Autodesk Inventor part; units mm, degrees
ref_plane "YZ Plane" through (0, 0, 0) normal (1, 0, 0) x (0, 1, 0)
ref_plane "XZ Plane" through (0, 0, 0) normal (0, 1, 0) x (-1, 0, 0)
ref_plane "XY Plane" through (0, 0, 0) normal (0, 0, 1) x (1, 0, 0)
sketch "Sketch1" plane through (0, 0, 0) normal (0, 1, 0) x (-1, 0, 0)
  line L0 (6.1765, 12) -> (-98.8235, 12)
  line L1 (-98.8235, 12) -> (-98.8235, -102)
  line L2 (-6.8235, 12) -> (-6.8235, 18)
  line L3 (-6.8235, 18) -> (6.1765, 18)
  line L4 (6.1765, 18) -> (6.1765, 12)
  line L5 (-98.8235, 12) -> (-98.8235, 18)
  line L6 (-98.8235, 18) -> (-85.8235, 18)
  line L7 (-85.8235, 18) -> (-85.8235, 12)
  line L8 (-98.8235, -102) -> (-85.8235, -87.8857)
  line L9 (-6.8235, -2.1143) -> (6.1765, 12)
  line L10 (-98.8235, -102) -> (-80.8235, -102)
  line L11 (6.1765, 12) -> (-80.8235, -102)
  point P0 (0, 0)
  point P1 (-96.8235, 18)
  point P2 (-96.8235, 18)
  dimension "d0" = 114
  dimension "d1" = 105
  dimension "d2" = 13
  dimension "d3" = 6
  dimension "d4" = 13
  dimension "d5" = 6
  dimension "d6" = 18
extrude "Extrusion1" add sketch "Sketch1" along normal blind 2
sketch "Sketch2" plane through (0, 2, 0) normal (0, 1, 0) x (1, 0, 0)
  line L0 (98.8235, 102) -> (80.8235, 102)
  line L1 (95.8235, 102) -> (87.8235, 102)
  line L2 (87.8235, 102) -> (87.8235, 92)
  line L3 (87.8235, 92) -> (95.8235, 92)
  line L4 (95.8235, 92) -> (95.8235, 102)
  line L5 (98.8235, -18) -> (98.8235, 102)
  point P0 (0, 0)
  dimension "d9" = 10
  dimension "d10" = 8
  dimension "d11" = 3
extrude "Extrusion2" add sketch "Sketch2" along normal blind 3
fillet "Fillet1" radius 4 2 edges at (87.8235, 5, -97) (95.8235, 5, -97)
sketch "Sketch3" plane through (0, 0, 0) normal (0, -1, 0) x (1, 0, 0)
  line L0 (87.8235, -102) -> (80.8235, -102)
  line L1 (87.8235, -102) -> (95.8235, -102)
  line L2 (95.8235, -102) -> (95.8235, -92)
  line L3 (95.8235, -92) -> (87.8235, -92)
  line L4 (87.8235, -92) -> (87.8235, -102)
  line L5 (98.8235, 18) -> (98.8235, -102)
  point P0 (0, 0)
  dimension "d16" = 10
  dimension "d17" = 8
  dimension "d18" = 3
extrude "Extrusion3" add sketch "Sketch3" along normal blind 3
fillet "Fillet3" radius 4 2 edges at (87.8235, -3, -97) (95.8235, -3, -97)
sketch "Sketch4" plane through (80.8235, 0, -102) normal (0, 0, -1) x (-1, 0, 0)
  arc A0 (-15, 0) -> (-11.127, -3) centre (-11.127, 1) ccw
  line L0 (-11.127, 4.8105) -> (-11.127, -3)
  circle A1 centre (-11.127, 1) radius 2.5
  point P0 (80.8235, 0)
  dimension "d25" = 5
extrude "Extrusion4" cut sketch "Sketch4" against normal blind 5
sketch "Sketch5" plane through (0, 2, 0) normal (0, 1, 0) x (1, 0, 0)
  line L0 (85.8235, -12) -> (85.8235, -18)
  line L1 (85.8235, -12) -> (98.8235, -12)
  line L2 (98.8235, -18) -> (98.8235, 102)
  circle A0 centre (92.3235, -12) radius 2.5
  point P0 (0, 0)
  dimension "d26" = 5
extrude "Extrusion5" cut sketch "Sketch5" against normal blind 2
sketch "Sketch6" plane through (0, 2, 0) normal (0, 1, 0) x (1, 0, 0)
  line L0 (-6.1765, -12) -> (-6.1765, -18)
  line L1 (6.8235, -18) -> (6.8235, -12)
  line L2 (-6.1765, -12) -> (6.8235, -12)
  circle A0 centre (0.3235, -12) radius 2.5
  point P0 (0, 0)
  dimension "d29" = 5
  dimension "d32" = 6.5
  dimension "d33" = 6
extrude "Extrusion6" cut sketch "Sketch6" against normal blind 2
equation "\"d23\" = d22"
properties part number "Triangle"
Input: part model. Units: mm. Frame: model coordinates. A direction names the side the tool comes from. Coordinates: 2 decimals unless noted, no trailing zeros. Loops run counter-clockwise (first coordinate to the right, second up) from the corner with the lowest first, then second, coordinate; pieces in that order, holes last. Notation, with made-up numbers: (-7, 59) - (36, 59) arc R18 cw to (36, 66) - close; hole circle Ø10 at (8.25, 3). An arc over 180 degrees is marked (long way). Answer in a Markdown table with one row per item. Add a question column.
Item 1: Contact query for flat-ended pins moving along their axis: P1, Ø1.5, axis at x = 90.5, y = 3.5, coming from the +Z side; P2, Ø4, axis at x = 0.32, z = 12, coming from the -Y side; P3, Ø1.5, axis at x = 58, z = -58.5, coming from the -Y side; P4, Ø12, axis at x = 63, z = -82, coming from the +Y side. Output: stop coordinate, or through.
Item 2: Section query A-A on z = -48. Return the cut outline in (x, y), then the cut area to 3 significant figures.
Item 3: Access query for faces 5 (the cylindrical face through (89.22, -2.14, -96.93)), 6 (the flat face through (92, -1, -92)), 7 (the cylindrical face through (89.566, 1.751, -99.535)). Directions: +Z, -Z, +X, -X, +Y, -Y. A direction counts if a zero-diameter tool reaches every point of the face in a straight line with its end or side. Return the directions, or none.
Item 4: Mould query, pull axis Y, two halves, no side actions, for faces 1 (the flat face through (70, 0, -41)), 2 (the cylindrical face through (94.43, 4.14, -96.93)), 3 (the flat face through (92, 3, -92)), 4 (the flat face through (92, 1, -97)). Classes: released by +Y, released by -Y, zero draft, split by the parting line, or undercut.
Item 5: Section query B-B on x = 59.5. Return the cut outline in (y, z), then the cut area to 3 significant figures.
Item 6: Line query: line 1 along Y through (x, z) = (69.5, -55); line 2 along X through (y, z) = (1, -100.15); line 3 along Z through (x, y) = (68.5, 0.75). Output: solid intervals per line, ascending. Write a range as [from, to].
Recorded:
| question | item | result |
|---|---|---|
| 1 | P1 | z = -92 |
| 1 | P2 | through |
| 1 | P3 | y = 0 |
| 1 | P4 | y = 2 |
| 2 | outline | (39.61, 0) - (98.82, 0) - (98.82, 2) - (39.61, 2) - close |
| 2 | area | 118 mm^2 |
| 3 | face 5 | +Z, -Z, -X, -Y |
| 3 | face 6 | +Z, +X, -X, -Y |
| 3 | face 7 | -Z |
| 4 | face 1 | released by -Y |
| 4 | face 2 | released by +Y |
| 4 | face 3 | zero draft |
| 4 | face 4 | undercut |
| 5 | outline | (0, -74.06) - (2, -74.06) - (2, 12) - (0, 12) - close |
| 5 | area | 172 mm^2 |
| 6 | line 1 | [0, 2] |
| 6 | line 2 | [79.41, 89.45], [94.45, 98.82] |
| 6 | line 3 | [-85.85, 12] |
